```python
from build123d import *

# Parameters (mm, degrees)
SKETCH2_W           = 72
SKETCH2_H           = 47
BOSS_EXTRUDE1_DEPTH = 3
FILLET1_R           = 2
SKETCH3_W           = 66.8
SKETCH3_H           = 41.8
SKETCH3_W_2         = 63.8
SKETCH3_H_2         = 38.8
BOSS_EXTRUDE2_DEPTH = 6
CUT_EXTRUDE1_DEPTH  = 6
SKETCH5_R           = 3.775
CUT_EXTRUDE2_DEPTH  = 10
CUT_EXTRUDE3_DEPTH  = 10


with BuildPart() as part:
    # Sketch2 → Boss-Extrude1 (new body)
    with BuildSketch(Plane(origin=(0, 0, 0), x_dir=(1, 0, 0), z_dir=(0, 1, 0))):
        with Locations((36, 23.5)):
            Rectangle(SKETCH2_W, SKETCH2_H)
    extrude(amount=BOSS_EXTRUDE1_DEPTH)

    # Fillet1
    fillet1_edges = [part.edges().sort_by_distance(p)[0] for p in [
        (0, 1.5, 0),
        (72, 1.5, 0),
        (72, 1.5, -47),
        (0, 1.5, -47),
    ]]
    fillet(fillet1_edges, radius=FILLET1_R)

    # Sketch3 → Boss-Extrude2 (add)
    with BuildSketch(Plane(origin=(0, 3, 0), x_dir=(1, 0, 0), z_dir=(0, 1, 0))):
        with Locations((36, 23.5)):
            Rectangle(SKETCH3_W, SKETCH3_H)
        with Locations((36, 23.5)):
            Rectangle(SKETCH3_W_2, SKETCH3_H_2, mode=Mode.SUBTRACT)
    extrude(amount=BOSS_EXTRUDE2_DEPTH)

    # Sketch4 → Cut-Extrude1 (cut)
    with BuildSketch(Plane.XZ):
        with BuildLine():
            Line((14, -9.5), (34, -9.5))
            ThreePointArc((34, -9.5), (36, -11.5), (34, -13.5))
            Line((34, -13.5), (14, -13.5))
            ThreePointArc((14, -13.5), (12, -11.5), (14, -9.5))
        make_face()
    extrude(amount=-CUT_EXTRUDE1_DEPTH, mode=Mode.SUBTRACT)

    # Sketch5 → Cut-Extrude2 (cut)
    with BuildSketch(Plane.XZ):
        with Locations(Location((24, -29.5, 0), (0, 0, 270))):
            Circle(SKETCH5_R)
    extrude(amount=-CUT_EXTRUDE2_DEPTH, mode=Mode.SUBTRACT)

    # Sketch7 → Cut-Extrude3 (cut)
    with BuildSketch(Plane.XZ):
        with BuildLine():
            Line((16.95, -28.05), (15.45, -27.75))
            add(Edge.make_bspline(
                [(15.45, -27.75), (15.16612192, -29.525922028), (15.45, -31.25)],
                knots=[0, 0, 0, 0.895638879, 0.895638879, 0.895638879], degree=2))
            Line((15.45, -31.25), (16.95, -30.95))
            add(Edge.make_bspline(
                [(16.95, -28.05), (16.795171073, -29.515331085), (16.95, -30.95)],
                knots=[0, 0, 0, 0.544466013, 0.544466013, 0.544466013], degree=2))
        make_face()
    extrude(amount=-CUT_EXTRUDE3_DEPTH, mode=Mode.SUBTRACT)


solid = part.part
```
The listing builds one solid part. Answer for the finished solid, in the listing's coordinates (mm). A direction names the side the tool comes from. Coordinates: 2 decimals unless noted, no trailing zeros. Loops run counter-clockwise (first coordinate to the right, second up) from the corner with the lowest first, then second, coordinate; pieces in that order, holes last. Notation, with made-up numbers: (19, 53.5) - (74, 53.5) arc R26 ccw to (74, 76.5) - close; hole circle Ø4 at (42.25, 63.5). An arc over 180 degrees is marked (long way). Use a Markdown table: item, result. Add a question column.
1) The part is cut by section D-D, the plane x = 50. Give the vertices of the cut face in (y, z), and give its area (3 significant figures).
2) For faces 4 (the cylindrical face through (36, 1.5, -11.5)), 5 (the flat face through (69.4, 6, -23)), 6 (the flat face through (36, 6, -42.9)), 7 (the flat face through (36, 6, -2.6)), 8 (the flat face through (36, 6, -44.4)), determine the directions among +Z, -Z, +X, -X, +Y, -Y from which every point of the face is accessible in a straight line to the end or side of a thin tool.
3) The part is cut by section A-A, the plane z = -11.5. Give the vertices of the cut face in (x, y).
4) The part is cut by section C-C, the plane y = 4.5. Give the vertices of the cut face in (x, z), and give its area (3 significant figures).
5) The mould has two halves that part along X. Classify faces 1 (the flat face through (2.6, 6, -23)), 2 (the cylindrical face through (21.703, 1.479, -26.504)), 3 (the flat face through (35, 0, -24)): released by +X, released by -X, zero draft, split by the parting line, or undercut.
6) Find the intervals of material crossed by line 1 (X direction, y = 1.4, z = -29.5) (3 decimals); line 2 (Z direction, x = 6, y = 4.75); line 3 (X direction, y = 6, z = -10.5), in increasing order.
7) Given pin 1 (3 mm diameter, centred on y = 5, z = -33, fed in from -X); pin 2 (5 mm diameter, centred on y = 7.5, z = -27.5, fed in from +X); pin 3 (5 mm diameter, centred on x = 32.5, y = 6.5, fed in from -Z), each flat-ended and moving along its own axis, determine where each tip first touches the part or whether it passes through.
8) The part is cut by section B-B, the plane x = 24. Give the vertices of the cut face in (y, z) (3 decimals).
Here are the results:
| question | item | result |
|---|---|---|
| 1 | outline | (0, -47) - (3, -47) - (3, -44.4) - (9, -44.4) - (9, -42.9) - (3, -42.9) - (3, -4.1) - (9, -4.1) - (9, -2.6) - (3, -2.6) - (3, 0) - (0, 0) - close |
| 1 | area | 159 mm^2 |
| 2 | face 4 | +Y, -Y |
| 2 | face 5 | +Z, -Z, +X, +Y |
| 2 | face 6 | +Y |
| 2 | face 7 | +Z, +X, -X, +Y |
| 2 | face 8 | -Z, +X, -X, +Y |
| 3 | outline | (0, 0) - (12, 0) - (12, 3) - (4.1, 3) - (4.1, 9) - (2.6, 9) - (2.6, 3) - (0, 3) - close; (36, 0) - (72, 0) - (72, 3) - (69.4, 3) - (69.4, 9) - (67.9, 9) - (67.9, 3) - (36, 3) - close |
| 4 | outline | (2.6, -44.4) - (69.4, -44.4) - (69.4, -2.6) - (2.6, -2.6) - close; hole (4.1, -42.9) - (67.9, -42.9) - (67.9, -4.1) - (4.1, -4.1) - close |
| 4 | area | 317 mm^2 |
| 5 | face 1 | released by -X |
| 5 | face 2 | undercut |
| 5 | face 3 | zero draft |
| 6 | line 1 | x = 0 to 15.308, 16.873 to 20.225, 27.775 to 72 |
| 6 | line 2 | z = -44.4 to -42.9, -4.1 to -2.6 |
| 6 | line 3 | x = 2.6 to 4.1, 67.9 to 69.4 |
| 7 | pin 1 | stops at x = 2.6 |
| 7 | pin 2 | stops at x = 69.4 |
| 7 | pin 3 | stops at z = -44.4 |
| 8 | outline | (0, -47) - (3, -47) - (3, -44.4) - (9, -44.4) - (9, -42.9) - (3, -42.9) - (3, -33.275) - (0, -33.275) - close; (0, -25.725) - (3, -25.725) - (3, -13.5) - (0, -13.5) - close; (0, -9.5) - (3, -9.5) - (3, -4.1) - (9, -4.1) - (9, -2.6) - (3, -2.6) - (3, 0) - (0, 0) - close |
